Drawing for the job (mm, zero at the part's lowest x, y, z). A direction names the side the tool comes from. Coordinates: 2 decimals unless noted, no trailing zeros. Order: outer loops, then holes, each group sorted by start corner. A loop starts at its lowest first (then second) coordinate and runs counter-clockwise, first axis right, second up.
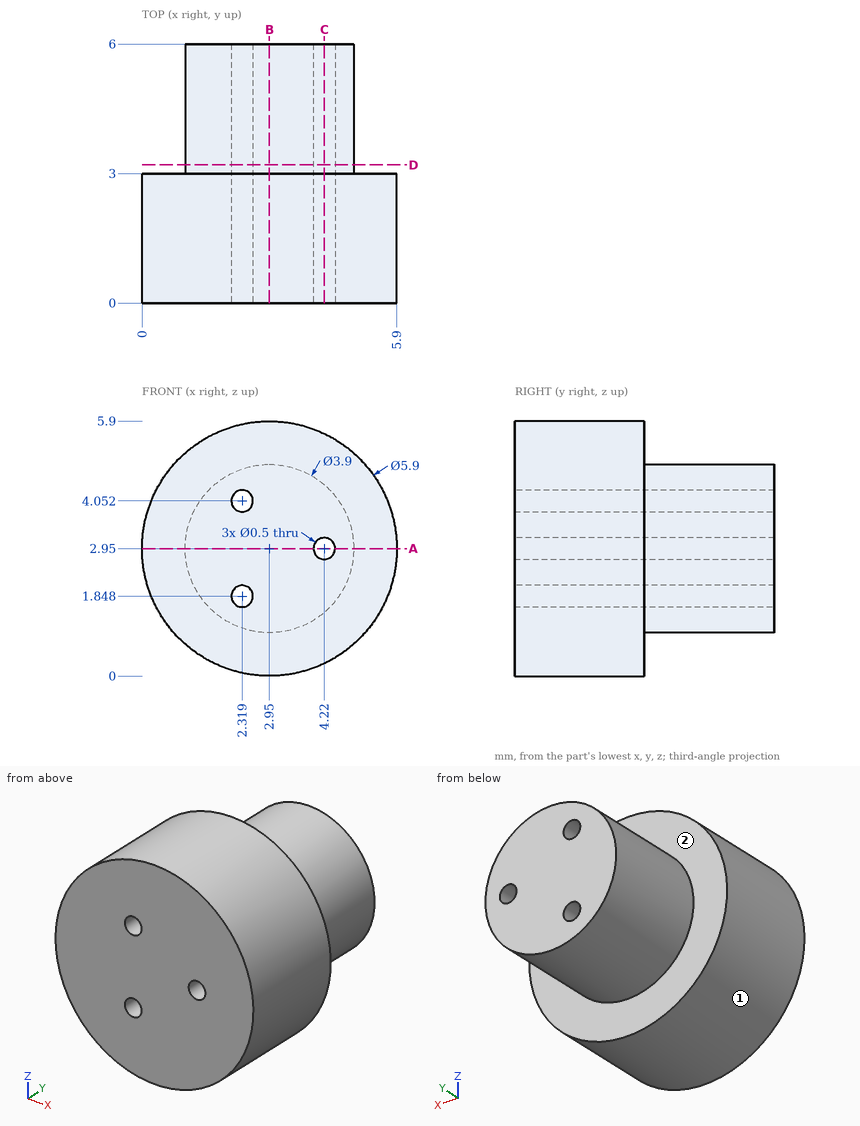
(1) Slice it at B-B, the plane x = 2.95. Give the cut face in (y, z), then the cut area to 3 significant figures.
(2) Probe line 1 (X direction, y = 1.5, z = 2.95); line 2 (Z direction, x = 2.45, y = 4.5) (1 decimal); line 3 (X direction, y = 3.15, z = 2.95). List the from-to ranges inside material, lowest first.
(3) Slice it at C-C, the plane x = 4.22. Give the cut face in (y, z).
(4) Slice it at D-D, the plane y = 3.2. Give the cut face in (x, z), then the cut area to 3 significant figures.
(5) Tool access for the marked faces 1 and 2: list every direction of +Z, -Z, +X, -X, +Y, -Y with a clear straight run to the whole face (end or side of a thin tool).
(6) Slice it at A-A, the plane z = 2.95. Give the cut face in (x, y).
(7) Drop a flat-ended pin along its axis: pin 1 (1.5 mm diameter, centred on y = 4, z = 3, fed in from -X). Give the stop position or say it passes through.
Here are the results:
1. outline: (0, 0) - (3, 0) - (3, 1) - (6, 1) - (6, 4.9) - (3, 4.9) - (3, 5.9) - (0, 5.9) - close
1. area: 29.4 mm2
2. line 1: x = 0 to 3.97, 4.47 to 5.9
2. line 2: z = 1.1 to 1.6, 2.1 to 3.8, 4.3 to 4.8
2. line 3: x = 1 to 3.97, 4.47 to 4.9
3. outline: (0, 0.29) - (3, 0.29) - (3, 1.47) - (6, 1.47) - (6, 2.7) - (0, 2.7) - close; (0, 3.2) - (6, 3.2) - (6, 4.43) - (3, 4.43) - (3, 5.61) - (0, 5.61) - close
4. outline: circle Ø3.9 at (2.95, 2.95); hole circle Ø0.5 at (2.32, 1.85); hole circle Ø0.5 at (2.32, 4.05); hole circle Ø0.5 at (4.22, 2.95)
4. area: 11.4 mm2
5. face 1: +Y, -Y
5. face 2: +Y
6. outline: (0, 0) - (3.97, 0) - (3.97, 6) - (1, 6) - (1, 3) - (0, 3) - close; (4.47, 0) - (5.9, 0) - (5.9, 3) - (4.9, 3) - (4.9, 6) - (4.47, 6) - close
7. pin 1: stops at x = 1
